Job drawing, mm, ordinate dimensions from the low corner. One solid piece. Round coordinates to 2 decimals unless told otherwise and drop trailing zeros. Loops run counter-clockwise (first coordinate to the right, second up) from the corner with the lowest first, then second, coordinate; pieces in that order, holes last. Notation, with made-up numbers: M 40.25,-32.75 L 56.25,-32.75 A15 cw 56.25,-4.75 Z; hole C -30,30 d9. An arc over 180 degrees is marked long. Use one line per item in the form item = value.
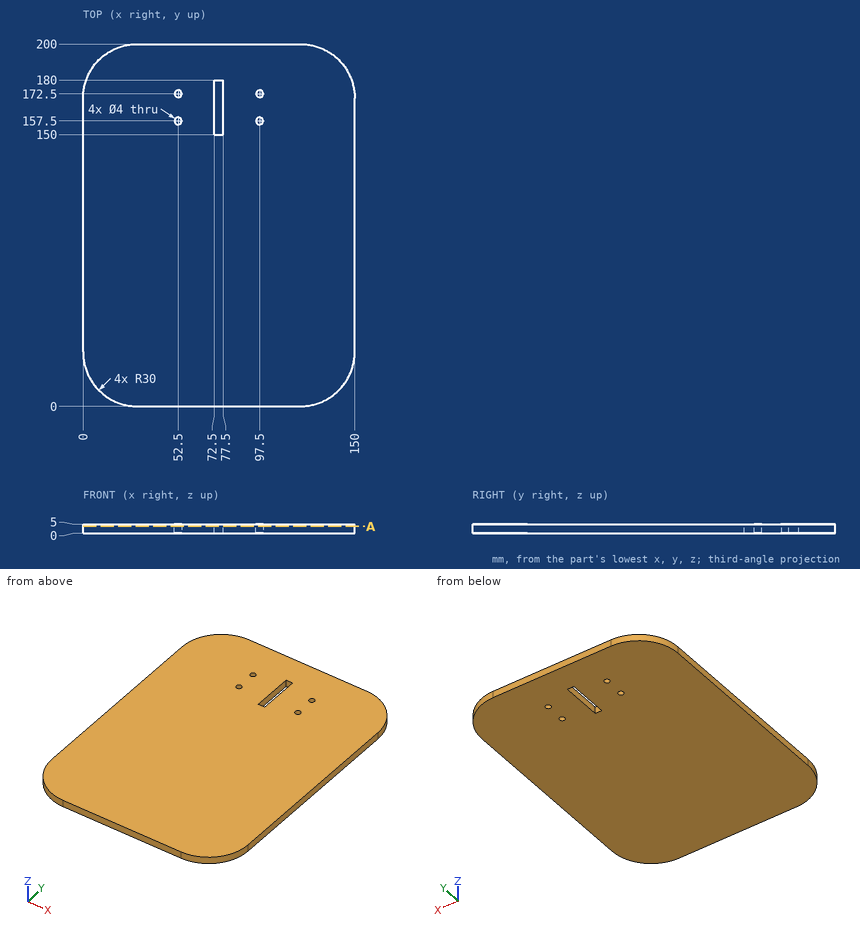
1. Cut at A-A on z = 3.9. Write the cut outline in (x, y).
Completed:
outline = M 0,30 A30 ccw 30,0 L 120,0 A30 ccw 150,30 L 150,170 A30 ccw 120,200 L 30,200 A30 ccw 0,170 Z; hole C 52.5,157.5 d4; hole C 52.5,172.5 d4; hole M 72.5,150 L 77.5,150 L 77.5,180 L 72.5,180 Z; hole C 97.5,157.5 d4; hole C 97.5,172.5 d4
2. Probe line 1 along X through (y, z) = (157.5, 1.65); line 2 along Y through (x, z) = (97.5, 3.05); line 3 along X through (y, z) = (153.5, 3.1). List the from-to ranges inside material, lowest first. Write a range as from..to.
Completed:
line_1 = 0..50.5, 54.5..72.5, 77.5..95.5, 99.5..150
line_2 = 0..155.5, 159.5..170.5, 174.5..200
line_3 = 0..72.5, 77.5..150
3. Drop a flat-ended pin along its axis: P1, Ø3.5, axis at x = 97.5, y = 157.5, coming from the -Z side (3 decimals). Give the stop position or say it passes through.
Completed:
P1 = through
